from build123d import *

# Parameters (mm, degrees)
SKETCH1_W           = 50.8
SKETCH1_H           = 68.2625
BOSS_EXTRUDE1_DEPTH = 7.9375
SKETCH2_W           = 50.8
SKETCH2_H           = 68.2625
SKETCH2_W_2         = 45.72
SKETCH2_H_2         = 63.1825
CUT_EXTRUDE1_DEPTH  = 2.54


with BuildPart() as part:
    # Sketch1 → Boss-Extrude1 (new body)
    with BuildSketch(Plane(origin=(0, 0, 0), x_dir=(1, 0, 0), z_dir=(0, 1, 0))):
        with Locations((25.4, 34.13125)):
            Rectangle(SKETCH1_W, SKETCH1_H)
    extrude(amount=BOSS_EXTRUDE1_DEPTH)

    # Sketch2 → Cut-Extrude1 (cut)
    with BuildSketch(Plane(origin=(0, 7.9375, 0), x_dir=(1, 0, 0), z_dir=(0, 1, 0))):
        with Locations((25.4, 34.13125)):
            Rectangle(SKETCH2_W, SKETCH2_H)
        with Locations((25.4, 34.13125)):
            Rectangle(SKETCH2_W_2, SKETCH2_H_2, mode=Mode.SUBTRACT)
    extrude(amount=-CUT_EXTRUDE1_DEPTH, mode=Mode.SUBTRACT)


solid = part.part
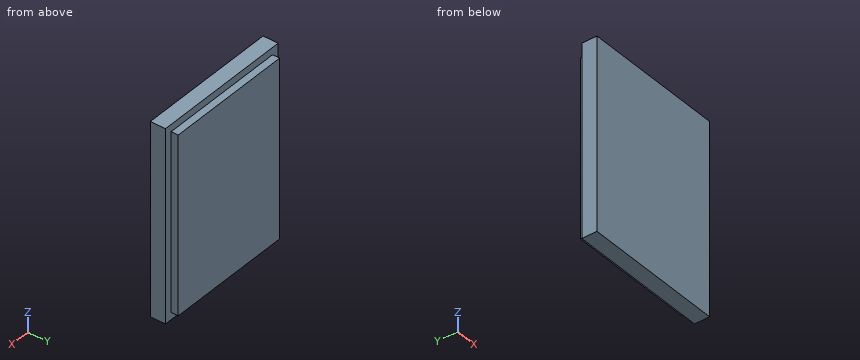
For this review, take the finished solid that the model builds, in its own axes (mm). Round coordinates to 2 decimals unless told otherwise and drop trailing zeros. Loops run counter-clockwise (first coordinate to the right, second up) from the corner with the lowest first, then second, coordinate; pieces in that order, holes last. Notation, with made-up numbers: (49.5, 42.5) - (80.5, 42.5) arc R13 ccw to (80.5, 46.5) - close; hole circle Ø2 at (20, 75). An arc over 180 degrees is marked (long way). Answer as CSV lines item,"result".
(1) Consider section A-A on x = 25. Give the boundary of the cut face in (y, z).
Checked values:
outline,"(0, -68.26) - (5.4, -68.26) - (5.4, -65.72) - (7.94, -65.72) - (7.94, -2.54) - (5.4, -2.54) - (5.4, 0) - (0, 0) - close"
(2) Consider section C-C on y = 7.25. Give the boundary of the cut face in (x, z).
Checked values:
outline,"(2.54, -65.72) - (48.26, -65.72) - (48.26, -2.54) - (2.54, -2.54) - close"
(3) Insertion check: P1, Ø0.8, axis at x = 36, y = 7, coming from the +Z side; P2, Ø2, axis at x = 26, y = 3, coming from the +Z side; P3, Ø0.8, axis at y = 6, z = -26.5, coming from the -X side; P4, Ø0.8, axis at x = 34, y = 6.5, coming from the -Z side. Each pin has a flat end and moves straight along its axis. Give the tip position at first contact, or say it passes through.
Checked values:
P1,"stops at z = -2.54"
P2,"stops at z = 0"
P3,"stops at x = 2.54"
P4,"stops at z = -65.72"
(4) Consider section B-B on z = -46. Give the boundary of the cut face in (x, y).
Checked values:
outline,"(0, 0) - (50.8, 0) - (50.8, 5.4) - (48.26, 5.4) - (48.26, 7.94) - (2.54, 7.94) - (2.54, 5.4) - (0, 5.4) - close"
(5) Wall thickness on line 1 (Y direction, x = 48.5, z = -38.5); line 2 (Z direction, x = 47, y = 6); line 3 (X direction, y = 5.75, z = -27): over which ranges is each line inside the solid? List them lowest first.
Checked values:
line 1,"y = 0 to 5.4"
line 2,"z = -65.72 to -2.54"
line 3,"x = 2.54 to 48.26"
